Drawing for the job (mm, zero at the part's lowest x, y, z). Coordinates: 2 decimals unless noted, no trailing zeros. Write each loop counter-clockwise with the first axis right and the second up, starting at its lowest first coordinate (ties: lowest second). Pieces come first, ordered by that corner, then holes. Notation, with made-up numbers: (-14.75, -9.5) -> (-6.75, -9.5) arc R31 ccw to (-6.75, 20.5) -> close; hole circle Ø6 at (23.5, 16). An arc over 180 degrees is marked (long way). Write item = value, one per line. Start each with the question number.
Q1. Pin check, flat tip, straight feed: P1, Ø10, axis at x = 22, z = 8, coming from the +Y side (3 decimals). Stop position of the tip, or through.
Q2. Probe line 1 (Z direction, x = 3, y = 49.5). List the from-to ranges inside material, lowest first.
Q3. Band-saw the part on A-A, the plane x = 39. List the corners of the cut face in (y, z).
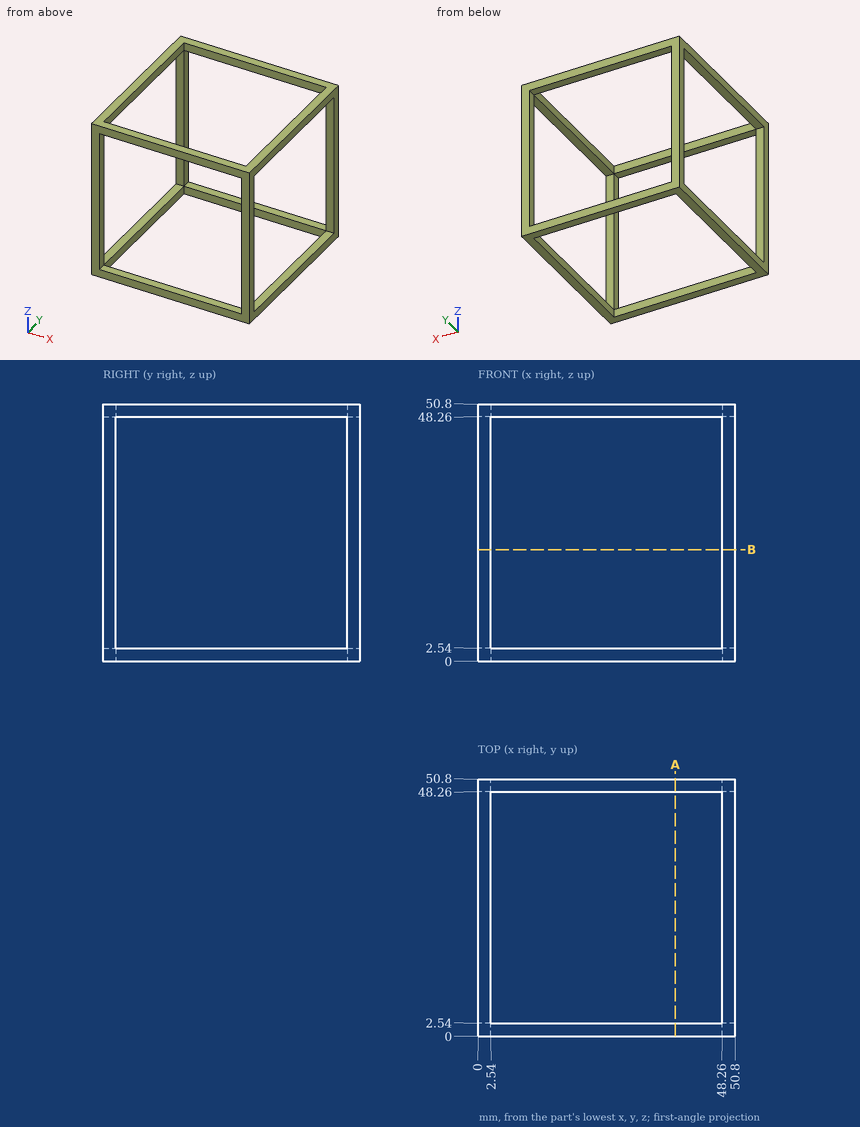
Ans:
q1.P1 = through
q2.line_1 = 0 to 2.54, 48.26 to 50.8
q3.outline = (0, 0) -> (2.54, 0) -> (2.54, 2.54) -> (0, 2.54) -> close; (0, 48.26) -> (2.54, 48.26) -> (2.54, 50.8) -> (0, 50.8) -> close; (48.26, 0) -> (50.8, 0) -> (50.8, 2.54) -> (48.26, 2.54) -> close; (48.26, 48.26) -> (50.8, 48.26) -> (50.8, 50.8) -> (48.26, 50.8) -> close
